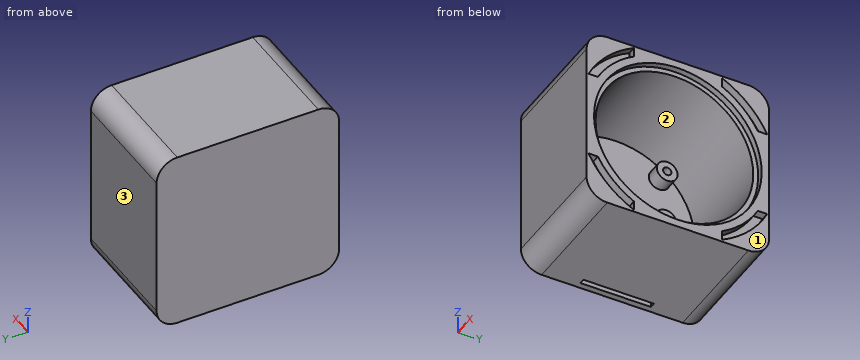
from build123d import *

# Parameters (mm, degrees)
SKETCH_1_W          = 44
SKETCH_1_H          = 44
EXTRUDE_1_DEPTH     = 1.5
SKETCH_2_R          = 2.5
SKETCH_2_R_2        = 1
EXTRUDE_2_DEPTH     = 3
SKETCH_3_R          = 2.5
SKETCH_3_R_2        = 1
EXTRUDE_3_DEPTH     = 3.5
SKETCH_4_W          = 44
SKETCH_4_H          = 44
SKETCH_4_R          = 19
EXTRUDE_4_DEPTH     = 27
CUT_EXTRUDE_START   = -1.5
SKETCH_5_R          = 20.2
SKETCH_5_R_2        = 19
CUT_EXTRUDE_1_DEPTH = 1.5
FILLET_2_R          = 5
CUT_EXTRUDE_START_2 = -10
SKETCH_10_W         = 1.3
SKETCH_10_H         = 17
CUT_EXTRUDE_5_DEPTH = 33.1930089
CUT_EXTRUDE_7_DEPTH = 2


with BuildPart() as part:
    # Sketch 1 → Extrude 1 (new body)
    with BuildSketch(Plane(origin=(0, 0, 0), x_dir=(0, 0, -1), z_dir=(1, 0, 0))):
        Rectangle(SKETCH_1_W, SKETCH_1_H)
    extrude(amount=EXTRUDE_1_DEPTH)

    # Sketch 2 → Extrude 2 (add)
    # profile 1 of 2: a face of its own
    with BuildSketch(Plane(origin=(1.5, 0, 0), x_dir=(0, 0, -1), z_dir=(1, 0, 0))):
        with Locations((0, -10.5)):
            Circle(SKETCH_2_R)
        with Locations(Location((0, -10.5, 0), (0, 0, 180))):
            Circle(SKETCH_2_R_2, mode=Mode.SUBTRACT)
    # profile 2 of 2: a face of its own
    with BuildSketch(Plane(origin=(1.5, 0, 0), x_dir=(0, 0, -1), z_dir=(1, 0, 0))):
        with Locations(Location((0, 10.5, 0), (0, 0, 180))):
            Circle(SKETCH_2_R)
        with Locations((0, 10.5)):
            Circle(SKETCH_2_R_2, mode=Mode.SUBTRACT)
    extrude(amount=EXTRUDE_2_DEPTH)

    # Sketch 3 → Extrude 3 (add)
    # profile 1 of 2: a face of its own
    with BuildSketch(Plane(origin=(1.5, 0, 0), x_dir=(0, 0, -1), z_dir=(1, 0, 0))):
        with Locations((-12.5, -10.5)):
            Circle(SKETCH_3_R)
        with Locations(Location((-12.5, -10.5, 0), (0, 0, 180))):
            Circle(SKETCH_3_R_2, mode=Mode.SUBTRACT)
    # profile 2 of 2: a face of its own
    with BuildSketch(Plane(origin=(1.5, 0, 0), x_dir=(0, 0, -1), z_dir=(1, 0, 0))):
        with Locations(Location((-12.5, 10.5, 0), (0, 0, 180))):
            Circle(SKETCH_3_R)
        with Locations((-12.5, 10.5)):
            Circle(SKETCH_3_R_2, mode=Mode.SUBTRACT)
    extrude(amount=EXTRUDE_3_DEPTH)

    # Sketch 4 → Extrude 4 (add)
    with BuildSketch(Plane(origin=(1.5, 0, 0), x_dir=(0, 0, -1), z_dir=(1, 0, 0))):
        Rectangle(SKETCH_4_W, SKETCH_4_H)
        Circle(SKETCH_4_R, mode=Mode.SUBTRACT)
    extrude(amount=EXTRUDE_4_DEPTH)

    # Sketch 5 → Cut-Extrude 1 (cut)
    with BuildSketch(Plane(origin=(28.5, 0, 0), x_dir=(0, 0, -1), z_dir=(1, 0, 0)).offset(CUT_EXTRUDE_START)):
        Circle(SKETCH_5_R)
        Circle(SKETCH_5_R_2, mode=Mode.SUBTRACT)
    extrude(amount=CUT_EXTRUDE_1_DEPTH, mode=Mode.SUBTRACT)

    # Fillet 2
    fillet_2_edges = [part.edges().sort_by_distance(p)[0] for p in [
        (14.25, -22, -22),
        (14.25, -22, 22),
        (14.25, 22, 22),
        (14.25, 22, -22),
    ]]
    fillet(fillet_2_edges, radius=FILLET_2_R)

    # Sketch 10 → Cut-Extrude 5 (cut, through all)
    with BuildSketch(Plane.XY.offset(CUT_EXTRUDE_START_2)):
        with Locations((2.15, 0)):
            Rectangle(SKETCH_10_W, SKETCH_10_H)
    extrude(amount=-CUT_EXTRUDE_5_DEPTH, mode=Mode.SUBTRACT)

    # Sketch 13 → Cut-Extrude 7 (cut)
    with BuildSketch(Plane(origin=(28.5, 0, 0), x_dir=(0, 0, -1), z_dir=(1, 0, 0))):
        with BuildLine():
            Line((-10.591663047, 21.536403458), (-10.591663047, 19.282548429))
            ThreePointArc((-10.591663047, 19.282548429), (-15.556349186, 15.556349186), (-19.282548429, 10.591663047))
            Line((-19.282548429, 10.591663047), (-21.536403458, 10.591663047))
            ThreePointArc((-21.536403458, 10.591663047), (-16.970562748, 16.970562748), (-10.591663047, 21.536403458))
        make_face()
        with BuildLine():
            Line((10.591663047, 21.536403458), (10.591663047, 19.282548429))
            ThreePointArc((10.591663047, 19.282548429), (15.556349186, 15.556349186), (19.282548429, 10.591663047))
            Line((19.282548429, 10.591663047), (21.536403458, 10.591663047))
            ThreePointArc((21.536403458, 10.591663047), (16.970562748, 16.970562748), (10.591663047, 21.536403458))
        make_face()
        with BuildLine():
            Line((-21.536403458, -10.591663047), (-19.282548429, -10.591663047))
            ThreePointArc((-19.282548429, -10.591663047), (-15.556349186, -15.556349186), (-10.591663047, -19.282548429))
            Line((-10.591663047, -19.282548429), (-10.591663047, -21.536403458))
            ThreePointArc((-10.591663047, -21.536403458), (-16.970562748, -16.970562748), (-21.536403458, -10.591663047))
        make_face()
        with BuildLine():
            Line((21.536403458, -10.591663047), (19.282548429, -10.591663047))
            ThreePointArc((19.282548429, -10.591663047), (15.556349186, -15.556349186), (10.591663047, -19.282548429))
            Line((10.591663047, -19.282548429), (10.591663047, -21.536403458))
            ThreePointArc((10.591663047, -21.536403458), (16.970562748, -16.970562748), (21.536403458, -10.591663047))
        make_face()
    extrude(amount=-CUT_EXTRUDE_7_DEPTH, mode=Mode.SUBTRACT)


solid = part.part
The listing builds one solid part. Answer for the finished solid, in the listing's coordinates (mm). Face numbers are marked on the shaded views. Coordinates: 2 decimals unless noted, no trailing zeros. Write each loop counter-clockwise with the first axis right and the second up, starting at its lowest first coordinate (ties: lowest second). Pieces come first, ordered by that corner, then holes. Notation, with made-up numbers: M 9.25,2.25 L 61.25,2.25 A7 ccw 61.25,11.25 Z; hole C 81.25,4.25 d11. An arc over 180 degrees is marked long. Write each question's results on one line, items separated by ' | '.
Item 1: The part is cut by section D-D on y = -18. Determine the outline of the cut face in (x, z), and give its area (3 significant figures).
Answer below:
outline: M 0,-21.9 L 28.5,-21.9 L 28.5,-15.87 L 26.5,-15.87 L 26.5,-12.65 L 28.5,-12.65 L 28.5,-9.17 L 27,-9.17 L 27,-6.08 L 1.5,-6.08 L 1.5,6.08 L 27,6.08 L 27,9.17 L 28.5,9.17 L 28.5,12.65 L 26.5,12.65 L 26.5,15.87 L 28.5,15.87 L 28.5,21.9 L 0,21.9 Z | area: 898 mm2
Item 2: The part is cut by section C-C on x = 16. Determine the outline of the cut face in (y, z).
Answer below:
outline: M -22,-17 A5 ccw -17,-22 L 17,-22 A5 ccw 22,-17 L 22,17 A5 ccw 17,22 L -17,22 A5 ccw -22,17 Z; hole C 0,0 d38
Item 3: For a pull along Y with two mould halves and no side action, classify the marked faces 1, 2 and 3 as released by +Y, released by -Y, zero draft, split by the parting line, or undercut.
Answer below:
face 1: zero draft | face 2: undercut | face 3: released by +Y
Item 4: The part is cut by section A-A on y = 0. Determine the outline of the cut face in (x, z), and give its area (4 significant figures).
Answer below:
outline: M 0,-22 L 1.5,-22 L 1.5,19 L 27,19 L 27,20.2 L 28.5,20.2 L 28.5,22 L 0,22 Z; M 2.8,-22 L 28.5,-22 L 28.5,-20.2 L 27,-20.2 L 27,-19 L 2.8,-19 Z | area: 220.5 mm2
Item 5: Consider probe 1 along Y at (x, z) = (3.6, 0); probe 2 along Y at (x, z) = (4.2, 12.5); probe 3 along Y at (x, z) = (3.5, 14). Determine where each line is inside the solid, lowest interval first. Write a range as [from, to].
Answer below:
probe 1: [-22, -19], [-13, -11.5], [-9.5, -8], [8, 9.5], [11.5, 13], [19, 22] | probe 2: [-22, -14.31], [-13, -11.5], [-9.5, -8], [8, 9.5], [11.5, 13], [14.31, 22] | probe 3: [-22, -12.85], [-12.5, -8.5], [8.5, 12.5], [12.85, 22]
Item 6: The part is cut by section B-B on z = 0. Determine the outline of the cut face in (x, y), and give its area (3 significant figures).
Answer below:
outline: M 0,-22 L 28.5,-22 L 28.5,-20.2 L 27,-20.2 L 27,-19 L 1.5,-19 L 1.5,-13 L 4.5,-13 L 4.5,-11.5 L 1.5,-11.5 L 1.5,-9.5 L 4.5,-9.5 L 4.5,-8 L 1.5,-8 L 1.5,8 L 4.5,8 L 4.5,9.5 L 1.5,9.5 L 1.5,11.5 L 4.5,11.5 L 4.5,13 L 1.5,13 L 1.5,19 L 27,19 L 27,20.2 L 28.5,20.2 L 28.5,22 L 0,22 Z | area: 242 mm2
Item 7: Given P1, Ø11.5, axis at y = -2.5, z = 1.5, coming from the +X side; P2, Ø2, axis at x = 27.5, z = -20, coming from the +Y side; P3, Ø3, axis at y = 10.5, z = 12.5, coming from the -X side; P4, Ø1.6, axis at x = 28, y = 21, coming from the -Z side, each flat-ended and moving along its own axis, determine where each tip first touches the part or whether it passes through.
Answer below:
P1: x = 4.5 | P2: y = 21.58 | P3: x = 0 | P4: z = -20.84
